For this review, take the finished solid that the model builds, in its own axes (mm). Face numbers are marked on the shaded views. A direction names the side the tool comes from. Round coordinates to 2 decimals unless told otherwise and drop trailing zeros. Order: outer loops, then holes, each group sorted by start corner. A loop starts at its lowest first (then second) coordinate and runs counter-clockwise, first axis right, second up. Notation, with made-up numbers: (77, 35) -> (102, 35) arc R15 ccw to (102, 39) -> close; hole circle Ø3 at (72.5, -0.5). An arc over 180 degrees is marked (long way). Answer in a Markdown table with one row per item.
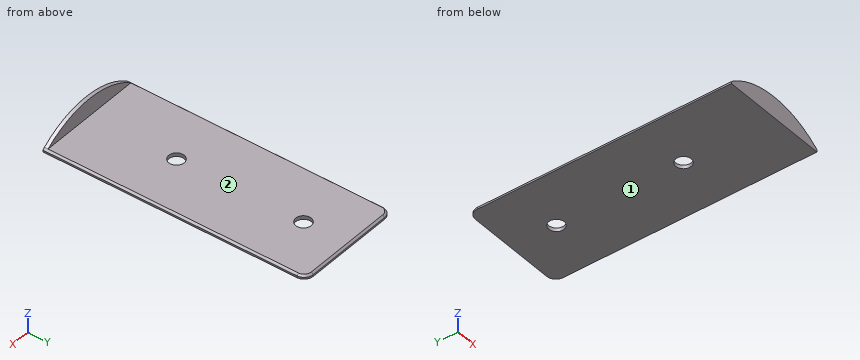
Solid Edge part; units mm, degrees
sketch "Sketch1" plane through (0, 0, 0) normal (0, 0, 1) x (1, 0, 0)
  circle A0 centre (60, 240) radius 8.5
  line L0 (120, 280) -> (120, 0)
  line L1 (120, 0) -> (0, 0)
  line L2 (0, 0) -> (0, 280)
  arc A1 (10, 290) -> (0, 280) centre (10, 280) ccw
  line L3 (10, 290) -> (110, 290)
  arc A2 (120, 280) -> (110, 290) centre (110, 280) ccw
  circle A3 centre (60, 100) radius 8.5
extrude "Protrusion1" add sketch "Sketch1" along normal blind 4
chamfer "Chaflán_1" distance 2 angle 45 5 edges at (0, 140, 4) (2.9289, 287.0711, 4) (60, 290, 4) (117.0711, 287.0711, 4) (120, 140, 4)
sketch "Sketch2" plane through (0, 0, 0) normal (0, 1, 0) x (-1, 0, 0)
  line L0 (-118, 4) -> (-2, 4)
  arc A0 (-2, 4) -> (-118, 4) centre (-60, -73.7496) ccw
extrude "ProtrusiónExtruida_4" add sketch "Sketch2" along normal blind 4
Q1. Take a section at B-B, the plane x = 60. Write out the cut boundary in (y, z).
Answer key:
| item | result |
|---|---|
| outline | (0, 0) -> (91.5, 0) -> (91.5, 4) -> (4, 4) -> (4, 23.25) -> (0, 23.25) -> close; (108.5, 0) -> (231.5, 0) -> (231.5, 4) -> (108.5, 4) -> close; (248.5, 0) -> (290, 0) -> (290, 2) -> (288, 4) -> (248.5, 4) -> close |
Q2. Take a section at D-D, the plane y = 28. Write out the cut boundary in (x, z), then the cut area to 3 significant figures.
Answer key:
| item | result |
|---|---|
| outline | (0, 0) -> (120, 0) -> (120, 2) -> (118, 4) -> (2, 4) -> (0, 2) -> close |
| area | 476 mm^2 |
Q3. Take a section at C-C, the plane x = 85. Write out the cut boundary in (y, z).
Answer key:
| item | result |
|---|---|
| outline | (0, 0) -> (290, 0) -> (290, 2) -> (288, 4) -> (4, 4) -> (4, 19.97) -> (0, 19.97) -> close |
Q4. Clearance check with flat-ended pins moving along their axes: pin 1 Ø1 at (x, z) = (61.5, 11) entering from +Y; pin 2 Ø4 at (x, y) = (79.5, 242.5) entering from +Z; pin 3 Ø3 at (x, y) = (17.5, 231.5) entering from -Z. State where each tip first meets the part, or that it passes through.
Answer key:
| item | result |
|---|---|
| pin 1 | stops at y = 4 |
| pin 2 | stops at z = 4 |
| pin 3 | stops at z = 0 |
Q5. Tool access review of the marked faces 1 and 2: name each direction out of +Z, -Z, +X, -X, +Y, -Y from which nothing blocks a thin tool from reaching the whole face with its end or side.
Answer key:
| item | result |
|---|---|
| face 1 | -Z, +X, -X, +Y, -Y |
| face 2 | +Z, +X, -X, +Y |
Q6. Take a section at A-A, the plane y = 100. Write out the cut boundary in (x, z).
Answer key:
| item | result |
|---|---|
| outline | (0, 0) -> (51.5, 0) -> (51.5, 4) -> (2, 4) -> (0, 2) -> close; (68.5, 0) -> (120, 0) -> (120, 2) -> (118, 4) -> (68.5, 4) -> close |
Q7. To check wall thickness, follow probe 1 along Y at (x, z) = (60, 2.5); probe 2 along Y at (x, z) = (91, 10). State the ranges of each line that lie inside material, in increasing order.
Answer key:
| item | result |
|---|---|
| probe 1 | y = 0 to 91.5, 108.5 to 231.5, 248.5 to 289.5 |
| probe 2 | y = 0 to 4 |
